Input: dimensioned drawing with shaded views. Units: mm. Origin: part minimum x, y, z. Give positions to 0.01 mm unless a question says otherwise; leave off trailing zeros. Order: outer loops, then holes, each group sorted by start corner. A loop starts at its lowest first (then second) coordinate and runs counter-clockwise, first axis right, second up. Notation, with made-up numbers: M 41,-32.75 L 54,-32.75 A17 cw 54,-13.75 Z; hole C -37,32 d2. An arc over 180 degrees is marked long. Answer in a Markdown table with one row per item. Add a question column.
(1) Section query A-A, the plane z = 1.35. Return loops of the section in (x, y).
(2) Pin query (flat end, axial travel): P1, Ø5, axis at x = 5.42, y = 4.52, coming from the +Z side; P2, Ø1.8, axis at x = 51.73, y = 27.23, coming from the -Z side. Return the tip coordinate at first contact, or that it passes through.
(3) Material intervals for line 1 along Y through (x, z) = (52, 0.95); line 2 along X through (y, z) = (27.5, 1.8); line 3 along Y through (x, z) = (51, 0.75), sorted ascending.
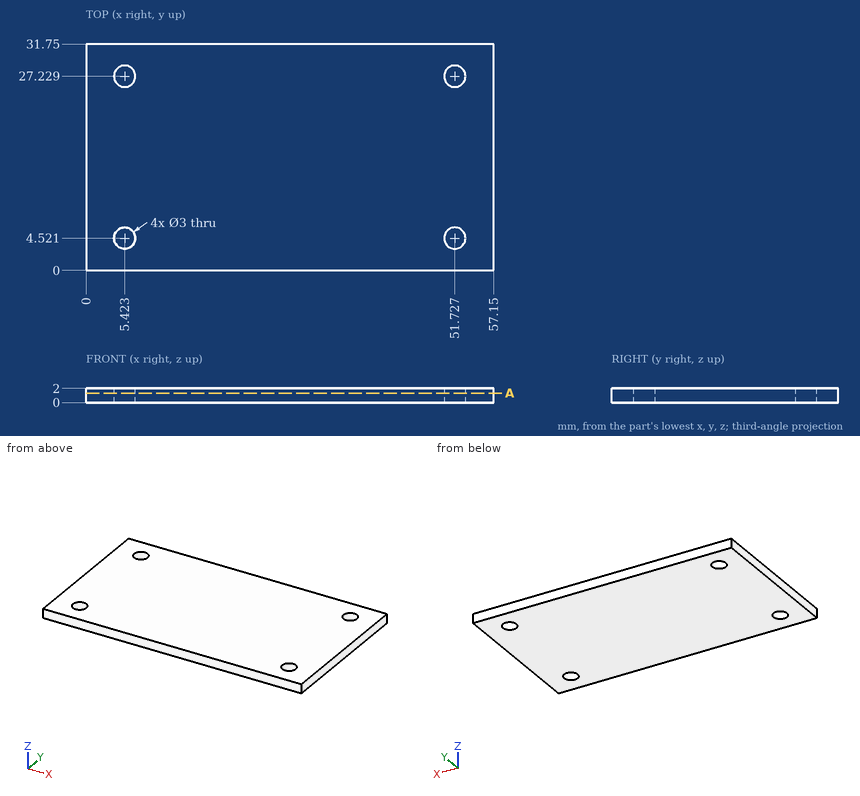
Values follow:
| question | item | result |
|---|---|---|
| 1 | outline | M 0,0 L 57.15,0 L 57.15,31.75 L 0,31.75 Z; hole C 5.42,4.52 d3; hole C 5.42,27.23 d3; hole C 51.73,4.52 d3; hole C 51.73,27.23 d3 |
| 2 | P1 | stops at z = 2 |
| 2 | P2 | passes through |
| 3 | line 1 | y = 0 to 3.05, 6 to 25.75, 28.7 to 31.75 |
| 3 | line 2 | x = 0 to 3.95, 6.9 to 50.25, 53.2 to 57.15 |
| 3 | line 3 | y = 0 to 3.21, 5.83 to 25.92, 28.54 to 31.75 |
